from build123d import *
from build123d.topology import SkipClean

# Parameters (mm, degrees)
SKETCH19_R           = 2.4
SKETCH19_R_2         = 3.65
BASE_DEPTH           = 10
CONNECTOR_DEPTH      = 36
SKETCH21_R           = 2.4
SKETCH21_R_2         = 1.35
THINPLATE_DEPTH      = 7
SPACER_START         = 6
SKETCH22_R           = 3
SKETCH22_R_2         = 1.35
SPACER_DEPTH         = 6
SHOCKHOLE_DEPTH      = 83.760860315
SKETCH25_R           = 2.4
SHOCKSCREWHOLE_DEPTH = 88.771065847
SKETCH26_R           = 4.3
BOLTMOUNT_DEPTH      = 8.6
NUTMOUNT_DEPTH       = 8


with BuildPart() as part:
    # Sketch19 → Base (new body)
    with BuildSketch(Plane(origin=(0, 0, 0), x_dir=(0, 0, -1), z_dir=(1, 0, 0))):
        with BuildLine():
            Line((-32, -8), (-2.8782e-05, -9.999989824))
            ThreePointArc((-2.8782e-05, -9.999989824), (5.231162179, -8.522585739), (8.916636561, -4.52691805))
            Line((8.916636561, -4.52691805), (31.214999285, 49.555458758))
            ThreePointArc((31.214999285, 49.555458758), (28.844541242, 56.814999285), (21.585000715, 54.444541242))
            Line((21.585000715, 54.444541242), (5.771017186, 23.295825861))
            Line((5.771017186, 23.295825861), (-22.627449378, 8))
            Line((-22.627449378, 8), (-32, 8))
            ThreePointArc((-32, 8), (-40, 0), (-32, -8))
        make_face()
        with Locations((26.4, 52)):
            Circle(SKETCH19_R, mode=Mode.SUBTRACT)
        with Locations((-2.8782e-05, 1.0176e-05)):
            Circle(SKETCH19_R_2, mode=Mode.SUBTRACT)
        with Locations((-32, 0)):
            Circle(SKETCH19_R, mode=Mode.SUBTRACT)
    extrude(amount=BASE_DEPTH)

    # Sketch20 → Connector (add)
    with BuildSketch(Plane(origin=(10, 0, 0), x_dir=(0, 0, -1), z_dir=(1, 0, 0))):
        with BuildLine():
            Line((-27.54952713, 8), (-32, 8))
            ThreePointArc((-32, 8), (-40, 0), (-32, -8))
            Line((-32, -8), (-27.086315803, -8.307103976))
            ThreePointArc((-27.086315803, -8.307103976), (-26.558475485, -7.826611078), (-26.485482069, -7.116568271))
            ThreePointArc((-26.485482069, -7.116568271), (-27.424283751, -0.187510507), (-26.580323996, 6.753737364))
            ThreePointArc((-26.580323996, 6.753737364), (-26.760140458, 7.613896312), (-27.54952713, 8))
        make_face()
        with BuildLine():
            Line((19.422577767, 50.185228792), (7.885841247, 27.461383049))
            ThreePointArc((7.885841247, 27.461383049), (14.036502787, 24.885542674), (19.422577767, 20.954157761))
            Line((19.422577767, 20.954157761), (29.406128946, 45.16823049))
            ThreePointArc((29.406128946, 45.16823049), (24.260347085, 47.370265615), (19.422577767, 50.185228792))
        make_face()
    extrude(amount=CONNECTOR_DEPTH)

    # Sketch21 → ThinPlate (add)
    with BuildSketch(Plane(origin=(46, 0, 0), x_dir=(0, 0, -1), z_dir=(1, 0, 0))):
        with BuildLine():
            Line((-22.627449378, 8), (-27.540134214, 8))
            Line((-27.540134214, 8), (-32, 8))
            ThreePointArc((-32, 8), (-40, 0), (-32, -8))
            Line((-32, -8), (-26.743480668, -8.328531082))
            Line((-26.743480668, -8.328531082), (-0.196731301, -9.987695968))
            ThreePointArc((-0.196731301, -9.987695968), (5.145129551, -8.567670884), (8.916636561, -4.52691805))
            Line((8.916636561, -4.52691805), (19.422577767, 20.954157761))
            Line((19.422577767, 20.954157761), (27.143694623, 39.680929602))
            Line((27.143694623, 39.680929602), (31.214999285, 49.555458758))
            ThreePointArc((31.214999285, 49.555458758), (28.844541242, 56.814999285), (21.585000715, 54.444541242))
            Line((21.585000715, 54.444541242), (17.595211042, 46.585874718))
            Line((17.595211042, 46.585874718), (5.771017186, 23.295825861))
            Line((5.771017186, 23.295825861), (0, 20.187472327))
            Line((0, 20.187472327), (-22.627449378, 8))
        make_face()
        with Locations((26.4, 52)):
            Circle(SKETCH21_R, mode=Mode.SUBTRACT)
        with Locations(Location((-32, 0, 0), (0, 0, 180))):
            Circle(SKETCH21_R, mode=Mode.SUBTRACT)
        with Locations((0.005188187, 0.010260161)):
            Circle(SKETCH21_R_2, mode=Mode.SUBTRACT)
    extrude(amount=THINPLATE_DEPTH)

    # Sketch22 → Spacer (add)
    with SkipClean():  # the faces are left unmerged after this step: merging them gives an invalid solid
        with BuildSketch(Plane.ZY.offset(-46).offset(SPACER_START)):
            with Locations(Location((-0.005188187, 0.010260161, 0), (0, 0, 180))):
                Circle(SKETCH22_R)
            with Locations((-0.005188187, 0.010260161)):
                Circle(SKETCH22_R_2, mode=Mode.SUBTRACT)
        extrude(amount=-SPACER_DEPTH)

    # Sketch23 → ShockHole (cut, through all)
    with SkipClean():  # the faces are left unmerged after this step: merging them gives an invalid solid
        with BuildSketch(Plane(origin=(0, 8, 0), x_dir=(1, 0, 0), z_dir=(0, 1, 0))):
            Polygon((19.5, -32), (19.5, -40.5), (36.5, -40.5), (36.5, -32), (36.5, -23.5), (19.5, -23.5), align=None)
        extrude(amount=-SHOCKHOLE_DEPTH, mode=Mode.SUBTRACT)

    # Sketch25 → ShockScrewHole (cut, through all)
    with BuildSketch(Plane.ZY):
        with Locations((32, 0)):
            Circle(SKETCH25_R)
    extrude(amount=-SHOCKSCREWHOLE_DEPTH, mode=Mode.SUBTRACT)

    # Sketch26 → BoltMount (cut)
    with SkipClean():  # the faces are left unmerged after this step: merging them gives an invalid solid
        with BuildSketch(Plane(origin=(53, 0, 0), x_dir=(0, 0, -1), z_dir=(1, 0, 0))):
            with Locations((-32, 0)):
                Circle(SKETCH26_R)
        extrude(amount=-BOLTMOUNT_DEPTH, mode=Mode.SUBTRACT)

    # Sketch27 → NutMount (cut)
    with SkipClean():  # the faces are left unmerged after this step: merging them gives an invalid solid
        with BuildSketch(Plane.ZY):
            Polygon((35.297994862, -2.894229297), (36.155473526, 1.409032684), (32.857478664, 4.303261981), (28.702005138, 2.894229297), (27.844526474, -1.409032684), (31.142521336, -4.303261981), align=None)
        extrude(amount=-NUTMOUNT_DEPTH, mode=Mode.SUBTRACT)


solid = part.part
The model under review builds one solid part; all positions refer to its coordinate system, in mm. A direction names the side the tool comes from. Give positions to 0.01 mm unless a question says otherwise; leave off trailing zeros. Write each loop counter-clockwise with the first axis right and the second up, starting at its lowest first coordinate (ties: lowest second). Pieces come first, ordered by that corner, then holes.
1. Draft analysis for pull direction Y (two halves, no side actions). For faces 5 (the flat face through (46, 50, -28)), 6 (the flat face through (3.94, 0.77, 28.28)), 7 (the cylindrical face through (41.183, -0.286, 27.423)), 8 (the cylindrical face through (49.451, -8.608, -5.078)), state which applies: +Y half, -Y half, draft (parallel to the pull), parting line (faces both ways), or undercut.
2. Wall thickness on L1, parallel to X at y = 4, z = 37; L2, parallel to X at y = -4, z = 10; L3, parallel to Y at x = 51, z = 32: over which ranges is each line inside the solid? List them lowest first.
3. Add section C-C, the plane y = 19. Write out the cut boundary in (x, z), plus the area to 3 significant figures.
4. Tool access review of faces 1 (the flat face through (3.94, -3.61, 33.19)), 2 (the flat face through (36.5, 0, 35)), 3 (the flat face through (7, 8, 28)), 4 (the cylindrical face through (27.748, 24.931, -13.955)): name each direction out of +Z, -Z, +X, -X, +Y, -Y from which nothing blocks a thin tool from reaching the whole face with its end or side.
5. Add section B-B, the plane y = 52. Write out the cut boundary in (x, z), plus the area to 3 significant figures.
6. Add section D-D, the plane x = 4. Write out the cut boundary in (y, z) (3 decimals).
7. For P1, Ø6, axis at x = 16.5, y = 27.5, coming from the -Z side; P2, Ø4.5, axis at x = 7.5, z = 28.5, coming from the +Y side; P3, Ø10, axis at x = 17.5, y = 37, coming from the -Z side, all flat-tipped, find the tip position at first contact; note any pin that passes through.
Worked answers:
1. face 5: draft
1. face 6: undercut
1. face 7: undercut
1. face 8: -Y half
2. L1: x = 0 to 19.5, 36.5 to 53
2. L2: x = 0 to 10, 46 to 53
2. L3: y = -8 to -4.3, 4.3 to 8
3. outline: (0, -18.62) - (10, -18.62) - (10, 2.2) - (0, 2.2) - close; (46, -18.62) - (53, -18.62) - (53, 2.2) - (46, 2.2) - close
3. area: 354 mm2
4. face 1: -X
4. face 2: +Z, -Z, +Y, -Y
4. face 3: +Z, +X, -X, +Y
4. face 4: +Z, -Y
5. outline: (0, -31.8) - (10, -31.8) - (10, -28.8) - (0, -28.8) - close; (0, -24) - (10, -24) - (10, -20.34) - (0, -20.34) - close; (46, -31.8) - (53, -31.8) - (53, -28.8) - (46, -28.8) - close; (46, -24) - (53, -24) - (53, -20.34) - (46, -20.34) - close
5. area: 113 mm2
6. outline: (-10, 0) arc R10 ccw to (-4.527, -8.917) - (49.555, -31.215) arc R5.4 ccw to (54.445, -21.585) - (23.296, -5.771) - (8, 22.627) - (8, 32) arc R8 ccw to (-8, 32) - close; hole (-4.303, 31.143) - (-1.409, 27.845) - (2.894, 28.702) - (4.303, 32.857) - (1.409, 36.155) - (-2.894, 35.298) - close; hole circle Ø7.3 at (0, 0); hole circle Ø4.8 at (52, -26.4)
7. P1: stops at z = -23.36
7. P2: stops at y = 8
7. P3: stops at z = -28.1
